```python
from build123d import *

# Parameters (mm, degrees)
F0_W     = 24.2662671953
F0_H     = 21.2902147323
F1_DEPTH = 25.4
F2_W     = 18.0781867821
F2_H     = 16.5515192784
F3_DEPTH = 12.7
F5_DEPTH = 12.7


with BuildPart() as f1:
    # F0 (on Top) → F1 (new body)
    with BuildSketch(Plane.XY):
        with Locations((-12.1331335977, 10.6451073661)):
            Rectangle(F0_W, F0_H)
        Polygon((-24.2662671953, 21.2902147323), (0, 21.2902147323), (0, 34.7969122231), (0, 35.7126183808), (-58.8342510164, 35.7126183808), (-54.7135621309, 31.82085976), (-58.8342510164, 29.76051718), (-24.2662671953, 29.76051718), align=None)
    extrude(amount=F1_DEPTH)

    # F2 (on face) → F3 (cut)
    with BuildSketch(Plane(origin=(0, 35.7126183808, 0), x_dir=(-1, 0, 0), z_dir=(0, 1, 0))):
        with Locations((12.5608363887, 12.9621129017)):
            Rectangle(F2_W, F2_H)
    extrude(amount=-F3_DEPTH, mode=Mode.SUBTRACT)

    # F4 (on face) → F5 (join)
    with BuildSketch(Plane.XY.offset(25.4)):
        with BuildLine():
            Line((-12.9212626108, 35.7126183808), (-13.2771370955, 35.7126183808))
            ThreePointArc((-13.2771370955, 35.7126183808), (-13.246046568, 35.3136187013), (-13.1263993339, 34.9317130788))
            ThreePointArc((-13.1263993339, 34.9317130788), (-12.1871466245, 23.7773669845), (-12.7422108084, 34.9574177981))
            ThreePointArc((-12.7422108084, 34.9574177981), (-12.8843245269, 35.3225499536), (-12.9212626108, 35.7126183808))
        make_face()
    extrude(amount=F5_DEPTH)


solid = f1.part
```
Design review of the part built by this model. Coordinates are the model's own, in mm. A direction names the side the tool comes from. Round coordinates to 2 decimals unless told otherwise and drop trailing zeros. Order: outer loops, then holes, each group sorted by start corner. A loop starts at its lowest first (then second) coordinate and runs counter-clockwise, first axis right, second up. Notation, with made-up numbers: M 40,-8 L 53,-8 A17 ccw 53,11 Z; hole C 15.25,-23.5 d10. An arc over 180 degrees is marked long. Put each result on its own line as item: value.
Q1. To check wall thickness, follow line 1 (Z direction, x = -16, y = 24.5); line 2 (X direction, y = 21, z = 16.5); line 3 (Y direction, x = -4, z = 7.5). State the ranges of each line that lie inside material, in increasing order.
Reported:
line 1: 0 to 4.69, 21.24 to 25.4
line 2: -24.27 to 0
line 3: 0 to 23.01
Q2. Consider section B-B (y = 33.5). State the section outline as (x, z) points.
Reported:
outline: M -56.49,0 L 0,0 L 0,25.4 L -8.79,25.4 L -8.79,38.1 L -16.33,38.1 L -16.33,25.4 L -56.49,25.4 Z; hole M -21.6,4.69 L -3.52,4.69 L -3.52,21.24 L -21.6,21.24 Z
Q3. Consider section C-C (x = -14). State the section outline as (y, z) points, and give its area (3 significant figures).
Reported:
outline: M 0,0 L 35.71,0 L 35.71,4.69 L 23.01,4.69 L 23.01,21.24 L 35.71,21.24 L 35.71,25.4 L 34.77,25.4 L 34.77,38.1 L 23.95,38.1 L 23.95,25.4 L 0,25.4 Z
area: 834 mm²
Q4. Insertion check: pin 1 Ø5 at (y, z) = (4, 23) entering from -X; pin 2 Ø4 at (x, z) = (-6.5, 28) entering from +Y; pin 3 Ø10 at (y, z) = (28, 9.5) entering from -X. Each pin has a flat end and moves straight along its axis. Give the tip position at first contact, or say it passes through.
Reported:
pin 1: x = -24.27
pin 2: y = 33.22
pin 3: x = -58.83
Q5. Draft analysis for pull direction Z (two halves, no side actions). For faces 4 (the face through (-12, 29, 4.686)), 5 (the face through (-12, 0, 13)), 6 (the face through (-13, 30, 38.1)), state which applies: released by +Z, released by -Z, zero draft, split by the parting line, or undercut.
Reported:
face 4: undercut
face 5: zero draft
face 6: released by +Z
Q6. Consider section D-D (y = 16.5). State the section outline as (x, z) points, and give its area (3 significant figures).
Reported:
outline: M -24.27,0 L 0,0 L 0,25.4 L -24.27,25.4 Z
area: 616 mm²
Q7. Machinability: for faces 1 (the face through (-42, 29.761, 13)), 2 (the face through (-12, 29, 21.238)), 3 (the face through (-56.8, 33.79, 12.52)), which of the approach directions +Z, -Z, +X, -X, +Y, -Y give a long, thin tool a straight path to every point of the face, cutting with its end or side? Answer none if there is none.
Reported:
face 1: +Z, -Z, -X, -Y
face 2: +Y
face 3: +Z, -Z, -X
Q8. Consider section A-A (z = 16). State the section outline as (x, y) points.
Reported:
outline: M -58.83,29.76 L -24.27,29.76 L -24.27,0 L 0,0 L 0,35.71 L -3.52,35.71 L -3.52,23.01 L -21.6,23.01 L -21.6,35.71 L -58.83,35.71 L -54.71,31.82 Z
